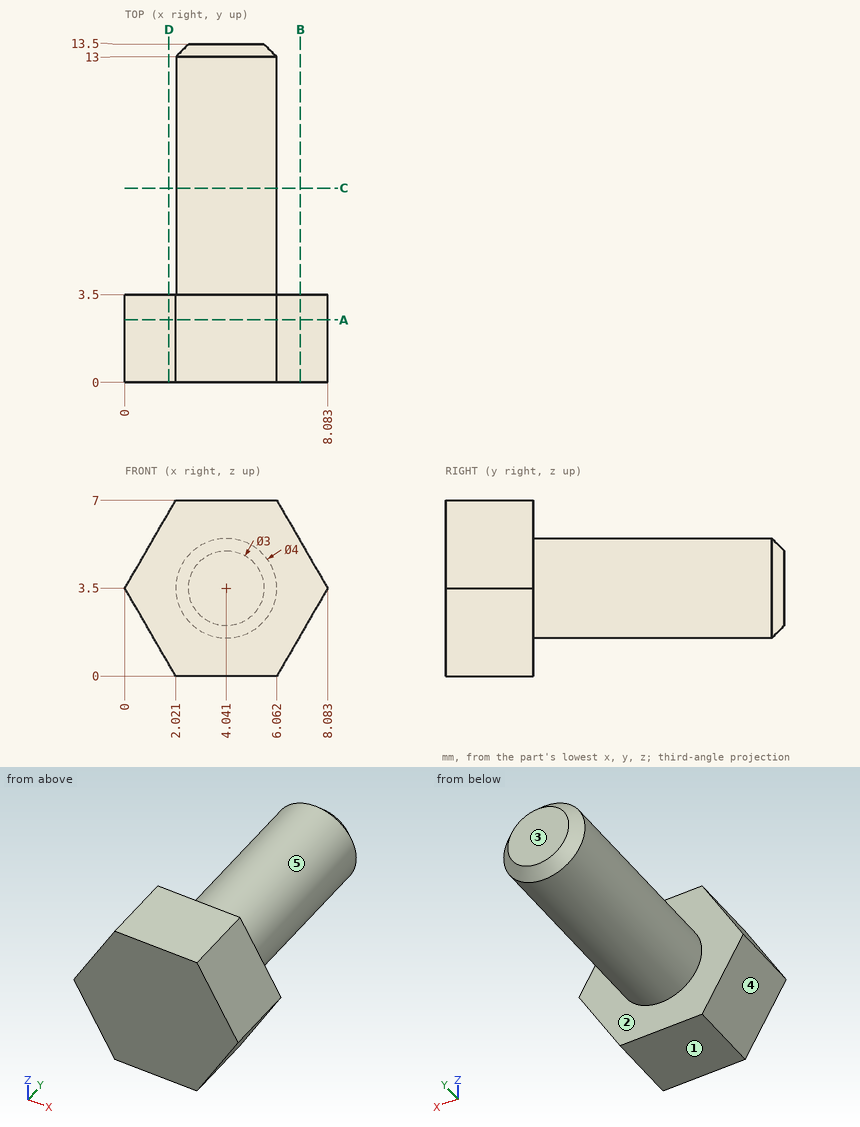
Part print with two shaded views. Sizes in mm from the minimum x, y, z corner. A direction names the side the tool comes from. Give positions to 0.01 mm unless a question says otherwise; leave off trailing zeros. Order: outer loops, then holes, each group sorted by start corner. A loop starts at its lowest first (then second) coordinate and runs counter-clockwise, first axis right, second up.
1) Saw through at C-C, the plane y = 7.75. Write the cut outline in (x, z).
2) Wall check: probe 1 along Y at (x, z) = (6.25, 3.5); probe 2 along Z at (x, y) = (4.75, 10); probe 3 along Y at (x, z) = (5.25, 2) (1 decimal). Give the ranges that are in metal, low to high.
3) Saw through at B-B, the plane x = 7. Write the cut outline in (y, z) (1 decimal).
4) Saw through at D-D, the plane x = 1.75. Write the cut outline in (y, z).
5) Mould opens along X. For the marked faces 3, 4 and 5 say: +X half, -X half, draft (parallel to the pull), parting line (faces both ways), or undercut.
6) Pin check, flat tips, straight feed: pin 1 (1.5 mm diameter, centred on x = 5, y = 7, fed in from -Z); pin 2 (2 mm diameter, centred on x = 1.5, y = 6, fed in from -Z) (1 decimal). Stop position of each tip, or through.
7) 3-axis set-ups, long thin cutter, end or side, ignore diameter. For the marked faces 1 and 2: which of +Z, -Z, +X, -X, +Y, -Y reach the whole face in a straight line?
8) Saw through at A-A, the plane y = 2.5. Write the cut outline in (x, z).
Computed:
1. outline: circle Ø4 at (4.04, 3.5)
2. probe 1: y = 0 to 3.5
2. probe 2: z = 1.63 to 5.37
2. probe 3: y = 0 to 13.1
3. outline: (0, 1.6) - (3.5, 1.6) - (3.5, 5.4) - (0, 5.4) - close
4. outline: (0, 0.47) - (3.5, 0.47) - (3.5, 6.53) - (0, 6.53) - close
5. face 3: draft
5. face 4: -X half
5. face 5: parting line
6. pin 1: stops at z = 1.51
6. pin 2: stops at z = 2.2
7. face 1: -Z, +X, -X, +Y, -Y
7. face 2: +Y
8. outline: (0, 3.5) - (2.02, 0) - (6.06, 0) - (8.08, 3.5) - (6.06, 7) - (2.02, 7) - close
